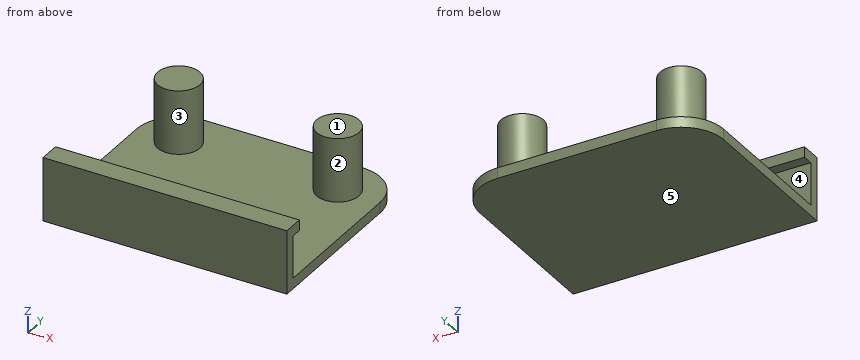
from build123d import *

# Parameters (mm, degrees)
EXTRUDE_THIN1_DEPTH = 115
FILLET1_R           = 20
SKETCH2_R           = 10
BOSS_EXTRUDE1_DEPTH = 30


with BuildPart() as part:
    # Sketch1 → Extrude-Thin1 (new body)
    with BuildSketch(Plane(origin=(0, 0, 0), x_dir=(0, 0, -1), z_dir=(1, 0, 0))):
        Polygon((0, 95), (0, 0), (-30, 0), (-30, 10), (-25, 10), (-25, 5), (-5, 5), (-5, 95), align=None)
    extrude(amount=EXTRUDE_THIN1_DEPTH)

    # Fillet1
    fillet1_edges = [part.edges().sort_by_distance(p)[0] for p in [
        (115, 95, 2.5),
        (0, 95, 2.5),
    ]]
    fillet(fillet1_edges, radius=FILLET1_R)

    # Sketch2 → Boss-Extrude1 (add)
    with BuildSketch(Plane.XY.offset(5)):
        with Locations(Location((20, 75, 0), (0, 0, 90))):
            Circle(SKETCH2_R)
        with Locations(Location((95, 75, 0), (0, 0, 90))):
            Circle(SKETCH2_R)
    extrude(amount=BOSS_EXTRUDE1_DEPTH)


solid = part.part
Read the model definition and answer for the solid it produces. Units are mm, in the model's axes. Face numbers are marked on the shaded views. A direction names the side the tool comes from. Round coordinates to 2 decimals unless told otherwise and drop trailing zeros. Order: outer loops, then holes, each group sorted by start corner. A loop starts at its lowest first (then second) coordinate and runs counter-clockwise, first axis right, second up.
1) The part is cut by section D-D on x = 22. Write down the section's boundary in (y, z).
2) The mould has two halves that part along X. Classify the marked faces 1 and 2: released by +X, released by -X, zero draft, split by the parting line, or undercut.
3) For the marked faces 3, 4 and 5, determine the directions among +Z, -Z, +X, -X, +Y, -Y from which every point of the face is accessible in a straight line to the end or side of a thin tool.
4) Straight lines are drawn through the part: L1, parallel to Y at x = 48, z = 10; L2, parallel to Y at x = 19.5, z = 4. For each, find the intervals that lie inside material, in ascending order.
5) The part is cut by section C-C on y = 60. Write down the section's boundary in (x, z).
6) The part is cut by section B-B on x = 59.5. Write down the section's boundary in (y, z), plus the area to 3 significant figures.
7) Flat-ended cylindrical pins translate along their axes: pin 1 (6 mm diameter, centred on x = 58.5, y = 79, fed in from +Z); pin 2 (4 mm diameter, centred on x = 67, z = 19.5, fed in from +Y); pin 3 (4 mm diameter, centred on x = 62.5, y = 70.5, fed in from -Z); pin 4 (2.5 mm diameter, centred on x = 64.5, z = 27, fed in from +Y). Find the tip coordinate at first contact, or state that the pin passes through.
8) The part is cut by section A-A on z = 6.5. Write down the section's boundary in (x, y), plus the area to 3 significant figures.
Resolved:
1. outline: (0, 0) - (95, 0) - (95, 5) - (84.8, 5) - (84.8, 35) - (65.2, 35) - (65.2, 5) - (5, 5) - (5, 25) - (10, 25) - (10, 30) - (0, 30) - close
2. face 1: zero draft
2. face 2: undercut
3. face 3: +Z
3. face 4: +X, -X
3. face 5: -Z, +X, -X, +Y, -Y
4. L1: y = 0 to 5
4. L2: y = 0 to 94.99
5. outline: (0, 0) - (115, 0) - (115, 5) - (0, 5) - close
6. outline: (0, 0) - (95, 0) - (95, 5) - (5, 5) - (5, 25) - (10, 25) - (10, 30) - (0, 30) - close
6. area: 625 mm2
7. pin 1: stops at z = 5
7. pin 2: stops at y = 5
7. pin 3: stops at z = 0
7. pin 4: stops at y = 10
8. outline: (0, 0) - (115, 0) - (115, 5) - (0, 5) - close; circle Ø20 at (20, 75); circle Ø20 at (95, 75)
8. area: 1,200 mm2
